The figure shows three views and two pictorial views of one solid part (mm, origin at its lowest corner). Answer the questions. Coordinates: 2 decimals unless noted, no trailing zeros. Loops run counter-clockwise (first coordinate to the right, second up) from the corner with the lowest first, then second, coordinate; pieces in that order, holes last.
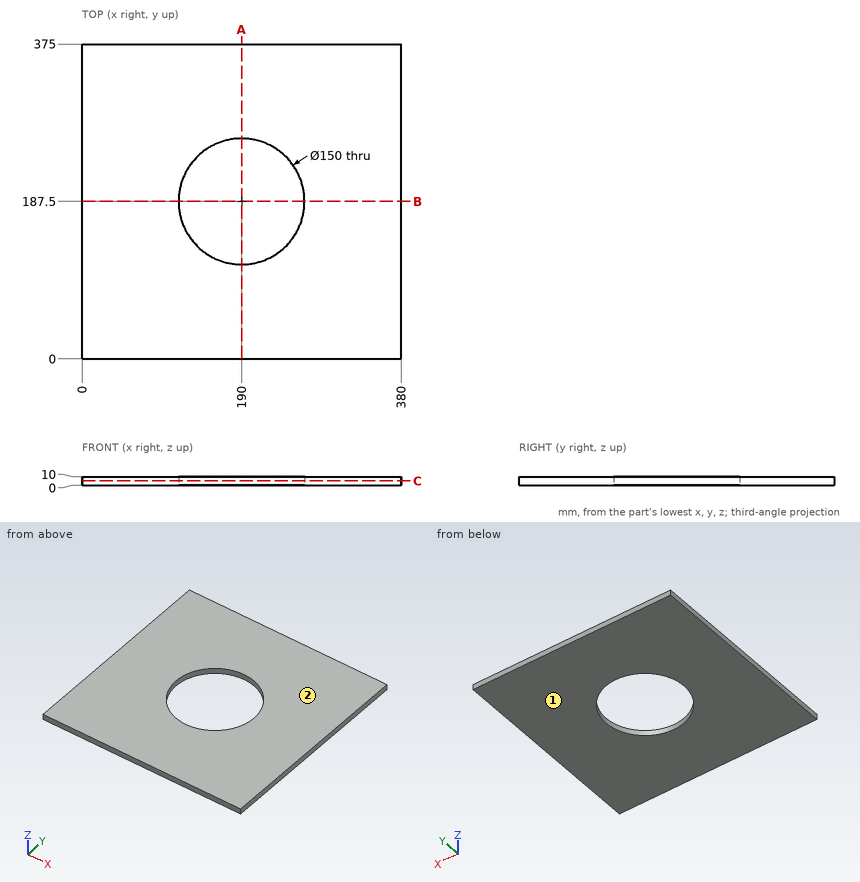
1. Determine the mould class of the marked faces 1 and 2 for opening direction Z: released by +Z, released by -Z, zero draft, split by the parting line, or undercut.
2. A cutting plane is placed at A-A, the plane x = 190. Give the vertices of the cut face in (y, z), then the cut area to 3 significant figures.
3. A cutting plane is placed at C-C, the plane z = 5.25. Give the vertices of the cut face in (x, y), then the cut area to 3 significant figures.
4. A cutting plane is placed at B-B, the plane y = 187.5. Give the vertices of the cut face in (x, z), then the cut area to 3 significant figures.
5. Straight lines are drawn through the part: probe 1 along Y at (x, z) = (190, 4.5); probe 2 along Y at (x, z) = (240, 1.5); probe 3 along X at (y, z) = (207, 8.75). For each, find the intervals that lie inside material, in ascending order.
Answers below:
1. face 1: released by -Z
1. face 2: released by +Z
2. outline: (0, 0) - (112.5, 0) - (112.5, 10) - (0, 10) - close; (262.5, 0) - (375, 0) - (375, 10) - (262.5, 10) - close
2. area: 2,250 mm2
3. outline: (0, 0) - (380, 0) - (380, 375) - (0, 375) - close; hole circle Ø150 at (190, 187.5)
3. area: 125,000 mm2
4. outline: (0, 0) - (115, 0) - (115, 10) - (0, 10) - close; (265, 0) - (380, 0) - (380, 10) - (265, 10) - close
4. area: 2,300 mm2
5. probe 1: y = 0 to 112.5, 262.5 to 375
5. probe 2: y = 0 to 131.6, 243.4 to 375
5. probe 3: x = 0 to 117.58, 262.42 to 380
